Solid Edge part; units mm, degrees
sketch "Sketch1" plane through (0, 0, 0) normal (0, -1, 0) x (1, 0, 0)
  line L0 (-21.15, 21.15) -> (21.15, 21.15)
  line L1 (21.15, 21.15) -> (21.15, -21.15)
  line L2 (21.15, -21.15) -> (-21.15, -21.15)
  line L3 (-21.15, -21.15) -> (-21.15, 21.15)
  dimension "D1" = 21.15
  dimension "D2" = 21.15
extrude "Protrusion1" add sketch "Sketch1" along normal mid plane 26
sketch "Sketch2" plane through (0, -13, 0) normal (0, -1, 0) x (1, 0, 0)
  circle A0 centre (0, 0) radius 2.5
extrude "Extrusionsausprägung_2" add sketch "Sketch2" along normal blind 24
hole "Bohrung_1" at (-15.5, -13, 15.5) direction (0, 1, 0) diameter 2.459 depth 10 tip angle 118 thread major 3 thread length 8
pattern_circular "Pattern1" count 4 over 360 about axis through (0, -13, 0) along (0, 1, 0) of "Bohrung_1"
chamfer "Fase_1" distance 5 angle 45 4 edges at (21.15, 0, 21.15) (-21.15, 0, 21.15) (21.15, 0, -21.15) (-21.15, 0, -21.15)
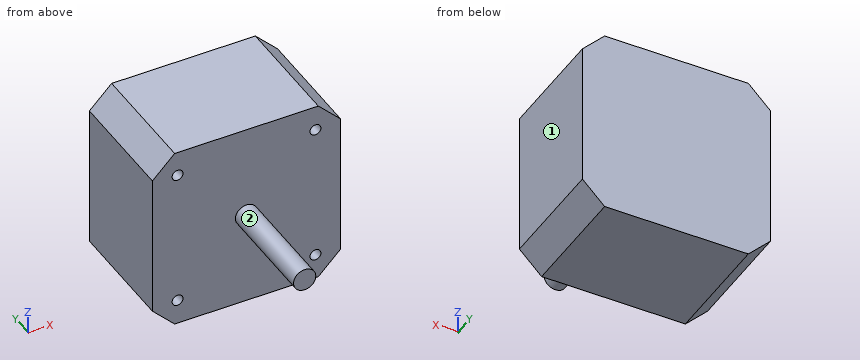
Geometry: final body of the model. Coordinates: model frame, mm. Face numbers are marked on the shaded views. A direction names the side the tool comes from. Coordinates: 2 decimals unless noted, no trailing zeros. Order: outer loops, then holes, each group sorted by start corner. A loop starts at its lowest first (then second) coordinate and runs counter-clockwise, first axis right, second up.
1) Section D-D (x = -18). Return loops of the section in (y, z).
Result sheet:
outline: (-13, -19.3) - (13, -19.3) - (13, 19.3) - (-13, 19.3) - close
2) Ray query, probe 1 along X at (y, z) = (-9.75, -15.5); probe 2 along X at (y, z) = (-7, -15). Return the intervals inside material, ascending.
Result sheet:
probe 1: x = -21.15 to -16.73, -14.27 to 14.27, 16.73 to 21.15
probe 2: x = -21.15 to -16.62, -14.38 to 14.38, 16.62 to 21.15
3) Set-up query: the marked faces 1 and 2. Return all of +Z, -Z, +X, -X, +Y, -Y with unobstructed straight access to the full face (end or side cutting, diameter ignored); none if empty.
Result sheet:
face 1: +Z, -Z, +X, +Y, -Y
face 2: -Y
4) Section C-C (z = 0). Return loops of the section in (x, y), then the cut area to 3 significant figures.
Result sheet:
outline: (-21.15, -13) - (-2.5, -13) - (-2.5, -37) - (2.5, -37) - (2.5, -13) - (21.15, -13) - (21.15, 13) - (-21.15, 13) - close
area: 1,220 mm2
5) Section B-B (y = 9). Return loops of the section in (x, z).
Result sheet:
outline: (-21.15, -16.15) - (-16.15, -21.15) - (16.15, -21.15) - (21.15, -16.15) - (21.15, 16.15) - (16.15, 21.15) - (-16.15, 21.15) - (-21.15, 16.15) - close
6) First-contact query: P1, Ø10, axis at y = -14.5, z = 6, coming from the -X side; P2, Ø5, axis at x = 1, y = -30.5, coming from the -Z side; P3, Ø1, axis at x = 9, z = 2.5, coming from the -Y side; P4, Ø2, axis at x = 15.5, z = 15.5, coming from the -Y side. Flat tips, straight axial feed; report the tip coordinate or a pass-through.
Result sheet:
P1: stops at x = -21.15
P2: stops at z = -2.5
P3: stops at y = -13
P4: stops at y = -2.86
7) Section A-A (y = -4). Return loops of the section in (x, z).
Result sheet:
outline: (-21.15, -16.15) - (-16.15, -21.15) - (16.15, -21.15) - (21.15, -16.15) - (21.15, 16.15) - (16.15, 21.15) - (-16.15, 21.15) - (-21.15, 16.15) - close; hole circle Ø2.46 at (-15.5, -15.5); hole circle Ø2.46 at (-15.5, 15.5); hole circle Ø2.46 at (15.5, -15.5); hole circle Ø2.46 at (15.5, 15.5)
